from build123d import *

# Parameters (mm, degrees)
SKETCH5_R            = 12.7
BOSS_EXTRUDE2_DEPTH  = 254
FILLET2_R            = 12.7
LPATTERN1_COUNT      = 2
LPATTERN1_PITCH      = 228.6
LPATTERN1_2_COUNT    = 2
LPATTERN1_2_PITCH    = 228.6
SKETCH6_R            = 12.7
BOSS_EXTRUDE3_DEPTH  = 114.3
LPATTERN2_COUNT      = 2
LPATTERN2_PITCH      = 228.6
LPATTERN2_COUNT_DIR2 = 2
LPATTERN2_PITCH_DIR2 = 228.6
SKETCH8_R            = 12.7
BOSS_EXTRUDE4_DEPTH  = 114.3
LPATTERN3_COUNT      = 2
LPATTERN3_PITCH      = 228.6
LPATTERN3_COUNT_DIR2 = 2
LPATTERN3_PITCH_DIR2 = 228.6


with BuildPart() as part:
    # Sketch5 → Boss-Extrude2 (new body)
    with BuildSketch(Plane(origin=(0, 0, 0), x_dir=(1, 0, 0), z_dir=(0, 1, 0))):
        with Locations(Location((-114.3, 114.3, 0), (0, 0, 270))):
            Circle(SKETCH5_R)
    extrude(amount=BOSS_EXTRUDE2_DEPTH)

    # Fillet2
    fillet2_edges = [part.edges().sort_by_distance(p)[0] for p in [
        (-114.3, 0, -127),
        (-114.3, 254, -127),
    ]]
    fillet(fillet2_edges, radius=FILLET2_R)


with BuildPart() as lpattern1_1:
    # LPattern1: pattern copy
    add(part.part.moved(Location(Vector(1, 0, 0) * (1 * LPATTERN1_PITCH))))


with BuildPart() as lpattern1_2_1:
    # LPattern1 2: pattern copy
    add(part.part.moved(Location(Vector(0, 0, 1) * (1 * LPATTERN1_2_PITCH))))



with BuildPart() as lpattern1_2_2:
    # LPattern1 2: pattern copy
    add(lpattern1_1.part.moved(Location(Vector(0, 0, 1) * (1 * LPATTERN1_2_PITCH))))


with BuildPart() as lpattern1_2_1_1:
    add(lpattern1_2_1.part)

    add(lpattern1_2_2.part)  # Boss-Extrude3 merges LPattern1 2_2
    # Sketch6 → Boss-Extrude3 (add, symmetric)
    with BuildSketch(Plane(origin=(0, 0, 0), x_dir=(0, 0, -1), z_dir=(1, 0, 0))):
        with Locations(Location((-114.3, 241.3, 0), (0, 0, 180))):
            Circle(SKETCH6_R)
    boss_extrude3 = extrude(amount=BOSS_EXTRUDE3_DEPTH, both=True)


with BuildPart() as part_1:
    add(part.part)

    add(lpattern1_1.part)  # LPattern2 merges LPattern1_1

    add(lpattern1_2_1_1.part)  # LPattern2 merges LPattern1 2_1
    # LPattern2: Boss-Extrude3 2 × 2
    with Locations(*[(0, -j * LPATTERN2_PITCH_DIR2, -i * LPATTERN2_PITCH) for i in range(LPATTERN2_COUNT) for j in range(LPATTERN2_COUNT_DIR2) if (i, j) != (0, 0)]):
        add(boss_extrude3)

    # Sketch8 → Boss-Extrude4 (add, symmetric)
    with BuildSketch(Plane.XY):
        with Locations(Location((-114.3, 241.3, 0), (0, 0, 180))):
            Circle(SKETCH8_R)
    boss_extrude4 = extrude(amount=BOSS_EXTRUDE4_DEPTH, both=True)

    # LPattern3: Boss-Extrude4 2 × 2
    with Locations(*[(i * LPATTERN3_PITCH, -j * LPATTERN3_PITCH_DIR2, 0) for i in range(LPATTERN3_COUNT) for j in range(LPATTERN3_COUNT_DIR2) if (i, j) != (0, 0)]):
        add(boss_extrude4)


solid = part_1.part
Check sheet for the modelled part. Datum: model origin and axes. Units: mm. Give positions to 0.01 mm unless a question says otherwise; leave off trailing zeros. Write each loop counter-clockwise with the first axis right and the second up, starting at its lowest first coordinate (ties: lowest second). Pieces come first, ordered by that corner, then holes. Notation, with made-up numbers: M 45,55.25 L 59,55.25 A32 cw 59,92.25 Z; hole C 14.25,75 d9. An arc over 180 degrees is marked long. Use one line per item in the form item = value.
(1) Material ranges on line 1 along X through (y, z) = (82, 116.5); line 2 along Y through (x, z) = (10, -105); line 3 along Y through (x, z) = (-22.5, 104.5), recorded low to high.
Answer block:
line_1 = -126.81 to -101.79, 101.79 to 126.81
line_2 = 4.05 to 21.35, 232.65 to 249.95
line_3 = 4.62 to 20.78, 233.22 to 249.38
(2) Section check C-C on z = -90. Record the boundary of the cut face in (x, y), plus the area to 3 significant figures.
Answer block:
outline = C -114.3,12.7 d25.4; C -114.3,241.3 d25.4; C 114.3,12.7 d25.4; C 114.3,241.3 d25.4
area = 2,030 mm2
(3) Section check B-B on x = 32. Record the boundary of the cut face in (y, z), plus the area to 3 significant figures.
Answer block:
outline = C 12.7,-114.3 d25.4; C 12.7,114.3 d25.4; C 241.3,-114.3 d25.4; C 241.3,114.3 d25.4
area = 2,030 mm2
(4) Section check A-A on y = 16.5. Record the boundary of the cut face in (x, z), plus the area to 3 significant figures.
Answer block:
outline = M -126.42,-110.5 A12.7 ccw -110.5,-126.42 L 110.5,-126.42 A12.7 ccw 126.42,-110.5 L 126.42,110.5 A12.7 ccw 110.5,126.42 L -110.5,126.42 A12.7 ccw -126.42,110.5 Z; hole M -102.18,-102.18 L 102.18,-102.18 L 102.18,102.18 L -102.18,102.18 Z
area = 22,100 mm2
